```python
from build123d import *

# Parameters (mm, degrees)
F0_W     = 3.5
F0_H     = 94
F1_DEPTH = 2.5
F2_R     = 1
F3_ANGLE = 30
F4_W     = 63.0289912224
F4_H     = 8.7771331891
F5_DEPTH = 25


with BuildPart() as f1:
    # F0 (on Front) → F1 (new body)
    with BuildSketch(Plane.XZ):
        with Locations((1.75, 47)):
            Rectangle(F0_W, F0_H)
    extrude(amount=F1_DEPTH)

    # F2
    f2_edges = [f1.edges().sort_by_distance(p)[0] for p in [
        (0, -1.25, 94),
        (3.5, -1.25, 94),
    ]]
    fillet(f2_edges, radius=F2_R)


with BuildPart() as f1_1:
    # F3: moved
    add(f1.part.rotate(Axis((0, -1.25, 0), (0, 1, 0)), F3_ANGLE))


with BuildPart() as f5:
    # F4 (on Front) → F5 (new body)
    with BuildSketch(Plane.XZ):
        with Locations((0.7424876094, -4.3885665946)):
            Rectangle(F4_W, F4_H)
    extrude(amount=F5_DEPTH)


with BuildPart() as f1_2:
    add(f1_1.part)

    # F6: cut F5
    add(f5.part, mode=Mode.SUBTRACT)


solid = f1_2.part
```
Here's how the part is built. I have some questions about the finished solid (model axes, mm). Give positions to 0.01 mm unless a question says otherwise; leave off trailing zeros. Write each loop counter-clockwise with the first axis right and the second up, starting at its lowest first coordinate (ties: lowest second). Pieces come first, ordered by that corner, then holes.
(1) Imagine slicing it at B-B, the plane z = 36. Write out the boundary of the cut face in (x, y).
Output values:
outline: (20.78, -2.5) - (24.83, -2.5) - (24.83, 0) - (20.78, 0) - close
(2) Imagine slicing it at A-A, the plane y = -1.45. Write out the boundary of the cut face in (x, z).
Output values:
outline: (0, 0) - (4.04, 0) - (49.53, 78.79) arc R1 ccw to (49.17, 80.16) - (47.87, 80.91) arc R1 ccw to (46.5, 80.54) - close
(3) Will these pins go through, and if not, where does the flat tip stop? pin 1 (10 mm diameter, centred on x = 18.5, z = 47, fed in from -Y); pin 2 (1.5 mm diameter, centred on y = -1, z = 65.5, fed in from -X); pin 3 (1 mm diameter, centred on x = 9.5, y = -0.5, fed in from +Z).
Output values:
pin 1: passes through
pin 2: stops at x = 37.38
pin 3: stops at z = 17.32
(4) Imagine slicing it at C-C, the plane x = 16. Write out the boundary of the cut face in (y, z).
Output values:
outline: (-2.5, 20.71) - (0, 20.71) - (0, 27.71) - (-2.5, 27.71) - close
(5) If I drill on L1, parallel to X at y = -0.85, z = 39; L2, parallel to X at y = -2.05, z = 63; L3, parallel to Z at x = 33, y = -0.55, over which ranges is the centre line in solid material (lowest first)?
Output values:
L1: x = 22.52 to 26.56
L2: x = 36.37 to 40.41
L3: z = 50.16 to 57.16
